Input: part model. Units: mm. Frame: model coordinates. A direction names the side the tool comes from. Give positions to 0.01 mm unless a question says otherwise; leave off trailing zeros. Loops run counter-clockwise (first coordinate to the right, second up) from the corner with the lowest first, then second, coordinate; pieces in that order, holes last.
from build123d import *

# Parameters (mm, degrees)
SKETCH1_W                      = 101.6
SKETCH1_H                      = 101.6
BOSS_EXTRUDE1_DEPTH            = 6.35
SKETCH2_W                      = 44.45
SKETCH2_H                      = 25.4
BOSS_EXTRUDE3_DEPTH            = 101.6
SKETCH4_W                      = 24.13
SKETCH4_H                      = 11.938
CUT_EXTRUDE1_DEPTH             = 101.6
SKETCH5_W                      = 43.18
SKETCH5_H                      = 38.1
BOSS_EXTRUDE4_DEPTH            = 101.6
SKETCH6_R                      = 10.795
CUT_EXTRUDE2_DEPTH             = 157.799568366
SKETCH7_W                      = 43.18
SKETCH7_H                      = 17.859873976
CUT_EXTRUDE3_DEPTH             = 157.799568366
CUT_EXTRUDE4_REACH             = 174.855
SKETCH8_W                      = 44.45
SKETCH8_H                      = 18.669
F_6_0_204_DIAMETER_HOLE1_D     = 5.1816
F_6_0_204_DIAMETER_HOLE1_DEPTH = 12.7
F_6_0_204_DIAMETER_HOLE1_TIP   = 1.556709692
F_6_0_204_DIAMETER_HOLE2_D     = 5.1816
F_6_0_204_DIAMETER_HOLE2_DEPTH = 12.7
F_6_0_204_DIAMETER_HOLE2_TIP   = 1.556709692
CUT_EXTRUDE5_START             = -38.1
SKETCH17_W                     = 43.18
SKETCH17_H                     = 1.905
CUT_EXTRUDE5_DEPTH             = 38.1
CUT_EXTRUDE6_START             = -25.4
SKETCH18_W                     = 44.45
SKETCH18_H                     = 1.905
CUT_EXTRUDE6_DEPTH             = 25.4


with BuildPart() as part:
    # Sketch1 → Boss-Extrude1 (new body)
    with BuildSketch(Plane.XY):
        with Locations((-50.8, 50.8)):
            Rectangle(SKETCH1_W, SKETCH1_H)
    extrude(amount=BOSS_EXTRUDE1_DEPTH)

    # Sketch2 → Boss-Extrude3 (add)
    with BuildSketch(Plane.XY.offset(6.35)):
        with Locations((-73.025, 76.2)):
            Rectangle(SKETCH2_W, SKETCH2_H)
    extrude(amount=BOSS_EXTRUDE3_DEPTH)

    # Sketch4 → Cut-Extrude1 (cut)
    with BuildSketch(Plane.XZ.offset(-63.5)):
        with Locations((-73.025, 89.281)):
            Rectangle(SKETCH4_W, SKETCH4_H)
    extrude(amount=-CUT_EXTRUDE1_DEPTH, mode=Mode.SUBTRACT)

    # Sketch5 → Boss-Extrude4 (add)
    with BuildSketch(Plane.XY.offset(6.35)):
        with Locations((-33.315999359, 32.041507513)):
            Rectangle(SKETCH5_W, SKETCH5_H)
    extrude(amount=BOSS_EXTRUDE4_DEPTH)

    # Sketch6 → Cut-Extrude2 (cut, through all)
    with BuildSketch(Plane(origin=(0, 51.091507513, 0), x_dir=(1, 0, 0), z_dir=(0, 1, 0))):
        with Locations(Location((-33.315999359, -90.17, 0), (0, 0, 270))):
            Circle(SKETCH6_R)
    extrude(amount=-CUT_EXTRUDE2_DEPTH, mode=Mode.SUBTRACT)

    # Sketch7 → Cut-Extrude3 (cut, through all)
    with BuildSketch(Plane(origin=(0, 51.091507513, 0), x_dir=(1, 0, 0), z_dir=(0, 1, 0))):
        with Locations((-33.315999359, -99.020063012)):
            Rectangle(SKETCH7_W, SKETCH7_H)
    extrude(amount=-CUT_EXTRUDE3_DEPTH, mode=Mode.SUBTRACT)

    # Sketch8 → Cut-Extrude4 (cut, up to next)
    with BuildSketch(Plane(origin=(0, 88.9, 0), x_dir=(1, 0, 0), z_dir=(0, 1, 0)), mode=Mode.PRIVATE) as cut_extrude4_sk1:
        with Locations((-73.025, -98.6155)):
            Rectangle(SKETCH8_W, SKETCH8_H)
    cut_extrude4_tool1 = extrude(cut_extrude4_sk1.sketch, amount=-CUT_EXTRUDE4_REACH, mode=Mode.PRIVATE) & part.part
    add(cut_extrude4_tool1.solids().sort_by_distance((-73.025, 88.9, 98.6155))[0], mode=Mode.SUBTRACT)

    # #6 (0.204) Diameter Hole1
    with Locations(Plane.XY.offset(90.090126024)):
        with Locations((-17.060294864, 22.643507513), (-17.313999359, 41.693507513), (-49.698703855, 41.439507513), (-49.698703855, 22.389507513)):
            Hole(F_6_0_204_DIAMETER_HOLE1_D / 2, depth=F_6_0_204_DIAMETER_HOLE1_DEPTH)
            with Locations((0, 0, -(F_6_0_204_DIAMETER_HOLE1_DEPTH + F_6_0_204_DIAMETER_HOLE1_TIP / 2))):  # 118° drill point
                Cone(0, F_6_0_204_DIAMETER_HOLE1_D / 2, F_6_0_204_DIAMETER_HOLE1_TIP, mode=Mode.SUBTRACT)

    # #6 (0.204) Diameter Hole2
    with Locations(Plane.XY.offset(89.281)):
        with Locations((-55.88, 82.55), (-55.88, 69.85), (-90.17, 82.55), (-90.17, 69.85)):
            Hole(F_6_0_204_DIAMETER_HOLE2_D / 2, depth=F_6_0_204_DIAMETER_HOLE2_DEPTH)
            with Locations((0, 0, -(F_6_0_204_DIAMETER_HOLE2_DEPTH + F_6_0_204_DIAMETER_HOLE2_TIP / 2))):  # 118° drill point
                Cone(0, F_6_0_204_DIAMETER_HOLE2_D / 2, F_6_0_204_DIAMETER_HOLE2_TIP, mode=Mode.SUBTRACT)

    # Sketch17 → Cut-Extrude5 (cut)
    with BuildSketch(Plane.XZ.offset(-12.991507513).offset(CUT_EXTRUDE5_START)):
        with Locations((-33.315999359, 89.137626024)):
            Rectangle(SKETCH17_W, SKETCH17_H)
    extrude(amount=CUT_EXTRUDE5_DEPTH, mode=Mode.SUBTRACT)

    # Sketch18 → Cut-Extrude6 (cut)
    with BuildSketch(Plane(origin=(0, 88.9, 0), x_dir=(1, 0, 0), z_dir=(0, 1, 0)).offset(CUT_EXTRUDE6_START)):
        with Locations((-73.025, -88.3285)):
            Rectangle(SKETCH18_W, SKETCH18_H)
    extrude(amount=CUT_EXTRUDE6_DEPTH, mode=Mode.SUBTRACT)


solid = part.part
(1) Ray query, probe 1 along X at (y, z) = (69.85, 83); probe 2 along Y at (x, z) = (-55.88, 80.5); probe 3 along Z at (x, y) = (-60, 92). Return the intervals inside material, ascending.
Values follow:
probe 1: x = -95.25 to -92.76, -87.58 to -58.47, -53.29 to -50.8
probe 2: y = 63.5 to 67.26, 72.44 to 79.96, 85.14 to 88.9
probe 3: z = 0 to 6.35
(2) Reachability of faces 4 (the flat face through (-52, 101.6, 3)), 5 (the cylindrical face through (-57.075, 67.552, 81.903)), 6 (the flat face through (-95.25, 76, 46)) from +Z, -Z, +X, -X, +Y, -Y: full face, straight path, thin tool, end or side. Return the list, or none.
Values follow:
face 4: +Z, -Z, +X, -X, +Y
face 5: +Z
face 6: +Z, -X, +Y, -Y
(3) Cut plane C-C (x = -26.5). Return the cut outline in (y, z).
Values follow:
outline: (0, 0) - (101.6, 0) - (101.6, 6.35) - (51.09, 6.35) - (51.09, 81.8) - (12.99, 81.8) - (12.99, 6.35) - (0, 6.35) - close
(4) Cut plane D-D (y = 15). Return the cut outline in (x, z) (3 decimals).
Values follow:
outline: (-101.6, 0) - (0, 0) - (0, 6.35) - (-11.726, 6.35) - (-11.726, 88.185) - (-22.705, 88.185) arc R10.795 cw to (-43.927, 88.185) - (-54.906, 88.185) - (-54.906, 6.35) - (-101.6, 6.35) - close
(5) Cut plane B-B (y = 87). Return the cut outline in (x, z).
Values follow:
outline: (-101.6, 0) - (0, 0) - (0, 6.35) - (-50.8, 6.35) - (-50.8, 87.38) - (-60.96, 87.38) - (-60.96, 83.31) - (-85.09, 83.31) - (-85.09, 87.38) - (-95.25, 87.38) - (-95.25, 6.35) - (-101.6, 6.35) - close
(6) Pin query (flat end, axial travel): pin 1 Ø8 at (x, y) = (-91.5, 77) entering from +Z; pin 2 Ø1.5 at (x, z) = (-82.5, 65) entering from +Y; pin 3 Ø1.5 at (x, z) = (-48, 20) entering from +Y; pin 4 Ø6 at (y, z) = (57, 55.5) entering from -X. Return the tip coordinate at first contact, or that it passes through.
Values follow:
pin 1: stops at z = 87.38
pin 2: stops at y = 88.9
pin 3: stops at y = 51.09
pin 4: passes through
(7) Cut plane A-A (z = 14.5). Return the cut outline in (x, y).
Values follow:
outline: (-95.25, 63.5) - (-50.8, 63.5) - (-50.8, 88.9) - (-95.25, 88.9) - close; (-54.91, 12.99) - (-11.73, 12.99) - (-11.73, 51.09) - (-54.91, 51.09) - close
(8) Mould query, pull axis X, two halves, no side actions, for faces 1 (the cylindrical face through (-33.107, 32.308, 79.377)), 2 (the flat face through (-54.906, 32, 47)), 3 (the flat face through (-34, 12.992, 47)). Classes: +X half, -X half, draft (parallel to the pull), parting line (faces both ways), or undercut.
Values follow:
face 1: undercut
face 2: -X half
face 3: draft
